Here's how the part is built. I have some questions about the finished solid (model axes, mm). Face numbers are marked on the shaded views. Coordinates: 2 decimals unless noted, no trailing zeros. Write each loop counter-clockwise with the first axis right and the second up, starting at its lowest first coordinate (ties: lowest second). Pieces come first, ordered by that corner, then holes.
Item 1: If we section it at C-C (z = 16.5): Please give me the cut outline in (x, y), then the cut area to 3 significant figures.
Item 2: If we section it at D-D (y = -33): Please give me the cut outline in (x, z).
Item 3: We'd pull the mould along X, two halves only. Please class the marked faces 1, 2 and 3: +X half, -X half, draft (parallel to the pull), parting line (faces both ways), or undercut.
Item 4: If we section it at B-B (x = -7.5): Please give me the cut outline in (y, z).
Item 5: I'm going to push flat-ended pins straight in: pin 1 Ø10 at (x, z) = (7, 15) entering from +Y; pin 2 Ø1.5 at (x, z) = (-26.5, 14.5) entering from +Y; pin 3 Ø3.5 at (x, y) = (0.46, 45.01) entering from +Z. Where does each tip first touch, or does it pass through?
Item 6: If I drill on line 1 (Y direction, x = 0, z = 14.5); line 2 (Z direction, x = 29, y = -37); line 3 (X direction, y = 12, z = 21.75), over which ranges is the centre line in solid material (lowest first)?
Item 7: If we section it at A-A (y = 0): Please give me the cut outline in (x, z), then the cut area to 3 significant figures.
from build123d import *

# Parameters (mm, degrees)
F0_R     = 37.846
F1_DEPTH = 25.4
F2_R     = 52.625625
F3_DEPTH = 1.5875
F4_R     = 35.798125
F5_DEPTH = 25.4
F6_R     = 1.2954
F7_DEPTH = 1.5885


with BuildPart() as f1:
    # F0 (on Top) → F1 (new body)
    with BuildSketch(Plane.XY):
        Circle(F0_R)
    extrude(amount=F1_DEPTH)

    # F2 (on Top) → F3 (join)
    with BuildSketch(Plane.XY):
        Circle(F2_R)
    extrude(amount=F3_DEPTH)

    # F4 (on Top) → F5 (cut, through all)
    with BuildSketch(Plane.XY):
        Circle(F4_R)
    extrude(amount=F5_DEPTH, mode=Mode.SUBTRACT)

    # F6 (on face) → F7 (cut, through all)
    with BuildSketch(Plane.XY.offset(1.5875)):
        with Locations((45.466, 0)):
            Circle(F6_R)
        with Locations((0.460375, -45.005625)):
            Circle(F6_R)
        with Locations((-44.54525, 0)):
            Circle(F6_R)
        with Locations((0.460375, 45.005625)):
            Circle(F6_R)
    extrude(amount=-F7_DEPTH, mode=Mode.SUBTRACT)


solid = f1.part
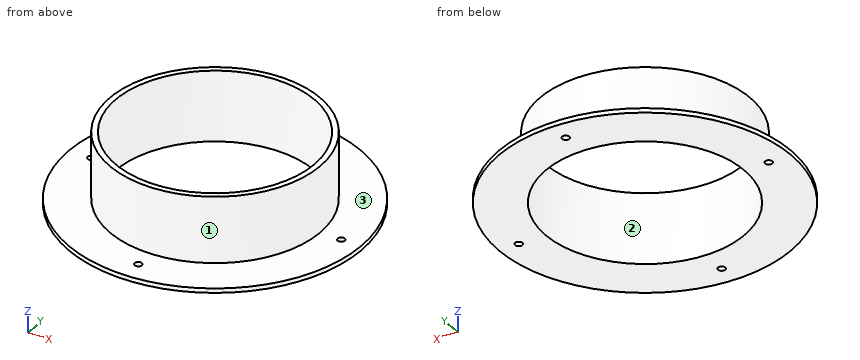
Answer list:
1. outline: circle Ø75.69 at (0, 0); hole circle Ø71.6 at (0, 0)
1. area: 474 mm2
2. outline: (-40.99, 0) - (-13.87, 0) - (-13.87, 25.4) - (-18.53, 25.4) - (-18.53, 1.59) - (-40.99, 1.59) - close; (13.87, 0) - (40.99, 0) - (40.99, 1.59) - (18.53, 1.59) - (18.53, 25.4) - (13.87, 25.4) - close
3. face 1: parting line
3. face 2: undercut
3. face 3: draft
4. outline: (-52.09, 0) - (-35, 0) - (-35, 25.4) - (-37.1, 25.4) - (-37.1, 1.59) - (-52.09, 1.59) - close; (35, 0) - (52.09, 0) - (52.09, 1.59) - (37.1, 1.59) - (37.1, 25.4) - (35, 25.4) - close
5. pin 1: stops at y = 37.79
5. pin 2: stops at y = 27.74
5. pin 3: stops at z = 1.59
6. line 1: y = -37.85 to -35.8, 35.8 to 37.85
6. line 2: z = 0 to 1.59
6. line 3: x = -35.89 to -33.73, 33.73 to 35.89
7. outline: (-52.63, 0) - (-45.84, 0) - (-45.84, 1.59) - (-52.63, 1.59) - close; (-43.25, 0) - (-35.8, 0) - (-35.8, 25.4) - (-37.85, 25.4) - (-37.85, 1.59) - (-43.25, 1.59) - close; (35.8, 0) - (44.17, 0) - (44.17, 1.59) - (37.85, 1.59) - (37.85, 25.4) - (35.8, 25.4) - close; (46.76, 0) - (52.63, 0) - (52.63, 1.59) - (46.76, 1.59) - close
7. area: 143 mm2
